```python
from build123d import *

# Parameters (mm, degrees)
SKETCH1_R           = 3.5
BOSS_EXTRUDE1_DEPTH = 0.5
SKETCH2_R           = 3.1
BOSS_EXTRUDE2_DEPTH = 3
SKETCH3_R           = 3.5
BOSS_EXTRUDE3_DEPTH = 9
SKETCH4_R           = 3.1
BOSS_EXTRUDE4_DEPTH = 6.6
FILLET1_R           = 0.5
BOSS_EXTRUDE5_DEPTH = 8.0772


with BuildPart() as part:
    # Sketch1 → Boss-Extrude1 (new body)
    with BuildSketch(Plane(origin=(0, 0, 0), x_dir=(1, 0, 0), z_dir=(0, 1, 0))):
        with Locations(Location((0, 0, 0), (0, 0, 270))):
            Circle(SKETCH1_R)
    extrude(amount=BOSS_EXTRUDE1_DEPTH)

    # Sketch2 → Boss-Extrude2 (add)
    with BuildSketch(Plane(origin=(0, 0.5, 0), x_dir=(1, 0, 0), z_dir=(0, 1, 0))):
        with Locations(Location((0, 0, 0), (0, 0, 270))):
            Circle(SKETCH2_R)
    extrude(amount=BOSS_EXTRUDE2_DEPTH)

    # Sketch3 → Boss-Extrude3 (add)
    with BuildSketch(Plane(origin=(0, 3.5, 0), x_dir=(1, 0, 0), z_dir=(0, 1, 0))):
        with Locations(Location((0, 0, 0), (0, 0, 270))):
            Circle(SKETCH3_R)
    extrude(amount=BOSS_EXTRUDE3_DEPTH)

    # Sketch4 → Boss-Extrude4 (add)
    with BuildSketch(Plane(origin=(0, 12.5, 0), x_dir=(1, 0, 0), z_dir=(0, 1, 0))):
        with Locations(Location((0, 0, 0), (0, 0, 270))):
            Circle(SKETCH4_R)
    extrude(amount=BOSS_EXTRUDE4_DEPTH)

    # Fillet1
    fillet1_edges = [part.edges().sort_by_distance(p)[0] for p in [
        (0, 19.1, -3.1),
    ]]
    fillet(fillet1_edges, radius=FILLET1_R)

    # Sketch5 → Boss-Extrude5 (add)
    with BuildSketch(Plane.XZ):
        with BuildLine():
            ThreePointArc((2.413, 0), (-1.060369493, 2.167529824), (-1.481061781, -1.905))
            Line((-1.481061781, -1.905), (1.481061781, -1.905))
            ThreePointArc((1.481061781, -1.905), (2.167529824, -1.060369493), (2.413, 0))
        make_face()
    extrude(amount=BOSS_EXTRUDE5_DEPTH)


solid = part.part
```
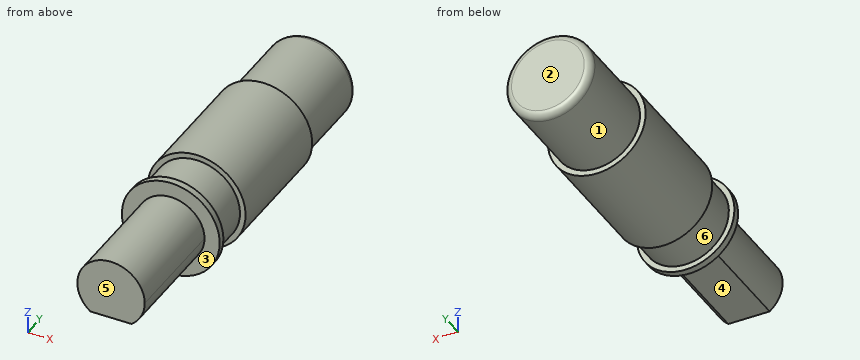
Work out the finished part from the listing and answer in its coordinate system (mm). Face numbers are marked on the shaded views. A direction names the side the tool comes from. Give positions to 0.01 mm unless a question says otherwise; leave off trailing zeros. Write each loop counter-clockwise with the first axis right and the second up, starting at its lowest first coordinate (ties: lowest second). Pieces come first, ordered by that corner, then holes. Notation, with made-up numbers: (74, 57) -> (132, 57) arc R21 ccw to (132, 61) -> close; hole circle Ø5 at (72, 64). An arc over 180 degrees is marked (long way). Write item = value, one per line.
Q1. Section C-C on y = -1.5 is taken. Determine the outline of the cut face in (x, z) (3 decimals).
Computed values:
outline = (-1.481, -1.905) -> (1.481, -1.905) arc R2.413 ccw (long way) to start
Q2. Section A-A on x = 0 is taken. Determine the outline of the cut face in (y, z) (3 decimals), and give its area (3 significant figures).
Computed values:
outline = (-8.077, -1.905) -> (0, -1.905) -> (0, -3.5) -> (0.5, -3.5) -> (0.5, -3.1) -> (3.5, -3.1) -> (3.5, -3.5) -> (12.5, -3.5) -> (12.5, -3.1) -> (18.6, -3.1) arc R0.5 ccw to (19.1, -2.6) -> (19.1, 2.6) arc R0.5 ccw to (18.6, 3.1) -> (12.5, 3.1) -> (12.5, 3.5) -> (3.5, 3.5) -> (3.5, 3.1) -> (0.5, 3.1) -> (0.5, 3.5) -> (0, 3.5) -> (0, 2.413) -> (-8.077, 2.413) -> close
area = 161 mm^2
Q3. Section D-D on y = 15.5 is taken. Determine the outline of the cut face in (x, z).
Computed values:
outline = circle Ø6.2 at (0, 0)
Q4. Consider line 1 along Y through (x, z) = (-1.5, 2.75); line 2 along Y through (x, z) = (2.25, -1); line 3 along Z through (x, y) = (0.5, 3.75). Determine where each line is inside the solid, lowest interval first.
Computed values:
line_1 = 0 to 0.5, 3.5 to 12.5
line_2 = 0 to 19.1
line_3 = -3.46 to 3.46
Q5. Flat-ended cylindrical pins translate along their axes: pin 1 Ø2 at (x, y) = (1.5, 16) entering from +Z; pin 2 Ø4 at (x, y) = (2.5, 7) entering from +Z; pin 3 Ø3.5 at (x, y) = (0, -5.5) entering from -Z (3 decimals). Find the tip coordinate at first contact, or state that the pin passes through.
Computed values:
pin_1 = 3.06
pin_2 = 3.46
pin_3 = -1.905
Q6. Section B-B on y = 9.25 is taken. Determine the outline of the cut face in (x, z), and give its area (3 significant figures).
Computed values:
outline = circle Ø7 at (0, 0)
area = 38.5 mm^2
Q7. For a pull along Y with two mould halves and no side action, classify the marked faces 4, 5 and 6 as pulls with the +Y half, pulls with the -Y half, needs draft (parallel to the pull), parting line crosses it, or undercut.
Computed values:
face_4 = needs draft
face_5 = pulls with the -Y half
face_6 = undercut
Q8. A tool of negligible diameter and unlimited length cuts with its end or side. For the marked faces 1, 2 and 3, from which of +Z, -Z, +X, -X, +Y, -Y can it reach the whole face along a straight path? Write none if from no direction.
Computed values:
face_1 = +Y
face_2 = +Z, -Z, +X, -X, +Y
face_3 = -Y
